The model under review builds one solid part; all positions refer to its coordinate system, in mm. Give positions to 0.01 mm unless a question says otherwise; leave off trailing zeros. Order: outer loops, then holes, each group sorted by start corner. A loop starts at its lowest first (then second) coordinate and runs counter-clockwise, first axis right, second up. Notation, with made-up numbers: M -19.75,13 L 33.25,13 A25 ccw 33.25,51 Z; hole C 72,38.5 d1. An arc over 180 degrees is marked long. One line per question, with ' | ' between items. Start each with the question number.
1. We need section A-A on y = 0. Write out the cut boundary in (x, z).
2. The part is to be moulded in two halves that separate along Y. For faces 1 (the face through (0, 0, 114.3)), 2 (the face through (-4.68, 4.29, 57.64)), 3 (the face through (0, -3.173, 59)), say which applies: +Y half, -Y half, draft (parallel to the pull), parting line (faces both ways), or undercut.
3. We need section B-B on x = 0. Write out the cut boundary in (y, z) (3 decimals).
4. Wall thickness on L1, parallel to Z at x = -2, y = -0.25; L2, parallel to Y at x = 0, z = 67; L3, parallel to Z at x = -5, y = 0.5: over which ranges is each line inside the solid? List them lowest first.
5. Insertion check: P1, Ø5, axis at x = 4, z = 63.5, coming from the -Y side. The pin has a flat end and moves straight along its axis. Give the tip position at first contact, or say it passes through.
6. We need section C-C on z = 64. Write out the cut boundary in (x, y).
```python
from build123d import *

# Parameters (mm, degrees)
F0_R     = 6.35
F1_DEPTH = 114.3
F2_R     = 2.54
F4_DEPTH = 12.7
F5_R     = 3.175
F6_DEPTH = 12.7


with BuildPart() as f1:
    # F0 (on Top) → F1 (new body)
    with BuildSketch(Plane.XY):
        Circle(F0_R)
    extrude(amount=F1_DEPTH)

    # F2
    f2_edges = [f1.edges().sort_by_distance(p)[0] for p in [
        (-6.35, 0, 0),
    ]]
    fillet(f2_edges, radius=F2_R)

    # F3 (on Right) → F4 (cut, symmetric)
    with BuildSketch(Plane.YZ):
        with BuildLine():
            Line((3.1722903245, 83.3166194451), (3.1723044783, 83.0546716063))
            ThreePointArc((3.1723044783, 83.0546716063), (3.1749999954, 83.1856456717), (3.1722903245, 83.3166194451))
        make_face()
        with BuildLine():
            Line((3.1749999954, 33.1680122005), (3.1723044783, 83.0546716063))
            Line((3.1723044783, 83.0546716063), (3.1722903245, 83.3166194451))
            ThreePointArc((3.1722903245, 83.3166194451), (-0.0080531428, 86.3604639044), (-3.1729147849, 83.3005252697))
            Line((-3.1729147849, 83.3005252697), (-3.1729147849, 83.0704229654))
            Line((-3.1729147849, 83.0704229654), (-3.1729147849, 33.2828917985))
            Line((-3.1729147849, 33.2828917985), (-3.1729147849, 33.0527894941))
            ThreePointArc((-3.1729147849, 33.0527894941), (0.0576207865, 29.9933635484), (3.1749999954, 33.1680122005))
        make_face()
        with BuildLine():
            Line((-3.1729147849, 83.0704229654), (-3.1729147849, 83.3005252697))
            ThreePointArc((-3.1729147849, 83.3005252697), (-3.175, 83.1854741175), (-3.1729147849, 83.0704229654))
        make_face()
        with BuildLine():
            ThreePointArc((-3.1729147849, 33.2828917985), (-3.175, 33.1678406463), (-3.1729147849, 33.0527894941))
            Line((-3.1729147849, 33.0527894941), (-3.1729147849, 33.2828917985))
        make_face()
    extrude(amount=F4_DEPTH, both=True, mode=Mode.SUBTRACT)

    # F5 (on Right) → F6 (cut, symmetric)
    with BuildSketch(Plane.YZ):
        with Locations((0, 105.5728718638)):
            Circle(F5_R)
    extrude(amount=F6_DEPTH, both=True, mode=Mode.SUBTRACT)


solid = f1.part
```
Entries:
1) outline: M -6.35,2.54 A2.54 ccw -3.81,0 L 3.81,0 A2.54 ccw 6.35,2.54 L 6.35,29.99 L -6.35,29.99 Z; M -6.35,86.36 L 6.35,86.36 L 6.35,102.4 L -6.35,102.4 Z; M -6.35,108.75 L 6.35,108.75 L 6.35,114.3 L -6.35,114.3 Z
2) face 1: draft | face 2: parting line | face 3: undercut
3) outline: M -6.35,2.54 A2.54 ccw -3.81,0 L 3.81,0 A2.54 ccw 6.35,2.54 L 6.35,114.3 L -6.35,114.3 Z; hole C 0,105.573 d6.35; hole M -3.173,33.283 A3.175 ccw long 3.175,33.168 L 3.172,83.055 A3.175 ccw long -3.173,83.07 Z
4) L1: z = 0 to 30, 86.35 to 102.41, 108.74 to 114.3 | L2: y = -6.35 to -3.17, 3.17 to 6.35 | L3: z = 0.31 to 30.03, 86.32 to 102.44, 108.71 to 114.3
5) P1: stops at y = -6.17
6) outline: M -5.5,-3.17 A6.35 ccw 5.5,-3.17 Z; M -5.5,3.17 L 5.5,3.17 A6.35 ccw Z
